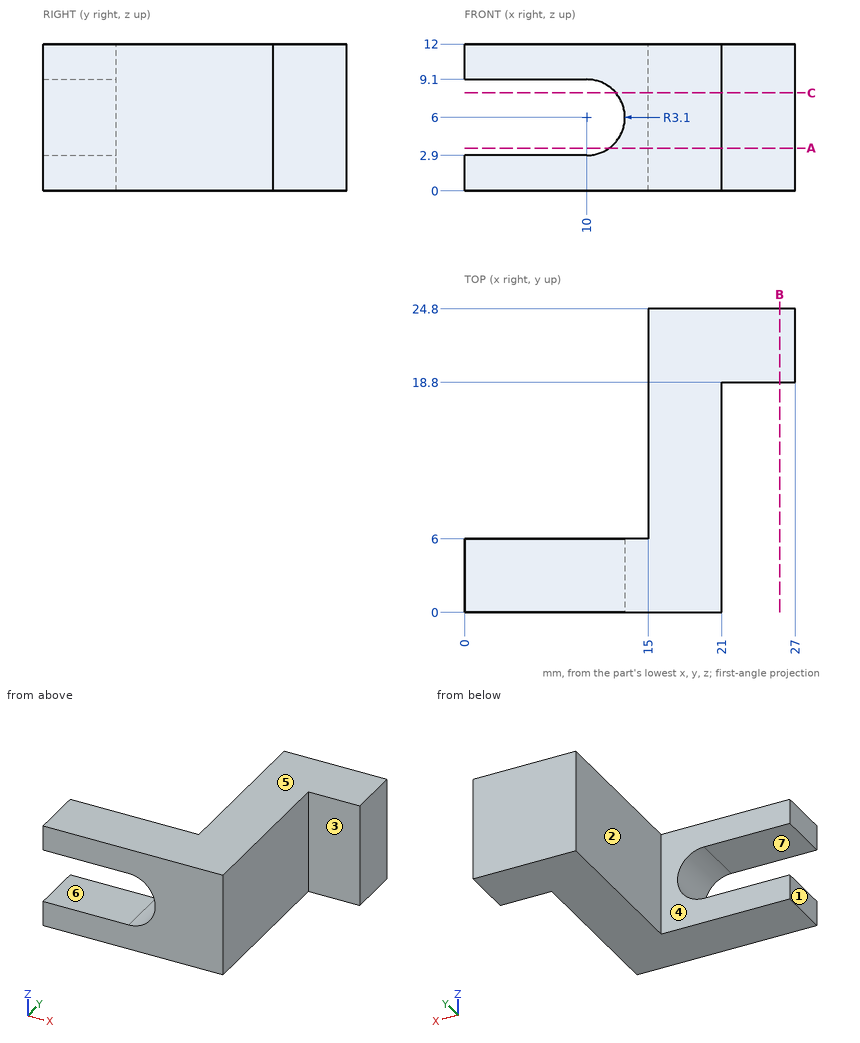
For this review, use the dimensioned drawing (mm, ordinates from the lowest corner) and the shaded views. A direction names the side the tool comes from. Round coordinates to 2 decimals unless told otherwise and drop trailing zeros. Order: outer loops, then holes, each group sorted by start corner. A loop starts at its lowest first (then second) coordinate and runs counter-clockwise, first axis right, second up. Notation, with made-up numbers: (69, -24.75) -> (126, -24.75) arc R21 ccw to (126, -14.75) -> close; hole circle Ø11 at (43, 55). An arc over 180 degrees is marked (long way). Write item = value, one per line. Start each with the question number.
Item 1: Clearance check with flat-ended pins moving along their axes: pin 1 Ø3.5 at (y, z) = (7, 6) entering from +X; pin 2 Ø5 at (x, z) = (24, 7.5) entering from -Y; pin 3 Ø6 at (x, z) = (4, 7.5) entering from +Y. State where each tip first meets the part, or that it passes through.
Item 2: Consider section C-C on z = 8. Write out the cut boundary in (x, y).
Item 3: Consider section A-A on z = 3.5. Write out the cut boundary in (x, y), plus the area to 3 significant figures.
Item 4: Mouldability with a two-part tool opening along Z and no side actions: class the marked faces 4, 5, 6 and 7 as released by +Z, released by -Z, zero draft, split by the parting line, or undercut.
Item 5: For the marked faces 1, 2 and 3, list the 3-axis set-ups (+Z, -Z, +X, -X, +Y, -Y) from which the entire face can be reached by the end or side of a thin tool; tool diameter is ignored.
Item 6: For line 1 along Z through (x, y) = (8, 3.75); line 2 along X through (y, z) = (2, 1); line 3 along X through (y, z) = (16.5, 4), list the stretches that pass through material, from the lowest coordinate up.
Item 7: Consider section B-B on x = 25.75. Write out the cut boundary in (y, z).
Conclusion:
q1.pin_1 = 21
q1.pin_2 = 18.8
q1.pin_3 = 6
q2.outline = (12.37, 0) -> (21, 0) -> (21, 18.8) -> (27, 18.8) -> (27, 24.8) -> (15, 24.8) -> (15, 6) -> (12.37, 6) -> close
q3.outline = (11.83, 0) -> (21, 0) -> (21, 18.8) -> (27, 18.8) -> (27, 24.8) -> (15, 24.8) -> (15, 6) -> (11.83, 6) -> close
q3.area = 204 mm2
q4.face_4 = zero draft
q4.face_5 = released by +Z
q4.face_6 = undercut
q4.face_7 = undercut
q5.face_1 = +Z, -Z, -X, +Y, -Y
q5.face_2 = +Z, -Z, -X, +Y
q5.face_3 = +Z, -Z, +X, -Y
q6.line_1 = 0 to 2.9, 9.1 to 12
q6.line_2 = 0 to 21
q6.line_3 = 15 to 21
q7.outline = (18.8, 0) -> (24.8, 0) -> (24.8, 12) -> (18.8, 12) -> close
